from build123d import *

# Parameters (mm, degrees)
F0_W     = 50.8
F0_H     = 38.1
F1_DEPTH = 25.4
F3_DEPTH = 50.8
F4_W     = 19.05
F4_H     = 12.7
F5_DEPTH = 19.05


with BuildPart() as f1:
    # F0 (on Front) → F1 (new body)
    with BuildSketch(Plane.XZ):
        with Locations((16.882635, 19.05)):
            Rectangle(F0_W, F0_H)
    extrude(amount=F1_DEPTH)

    # F2 (on face) → F3 (cut)
    with BuildSketch(Plane.YZ.offset(42.282635)):
        with BuildLine():
            Line((-25.4, 38.1), (-25.4, 12.7))
            ThreePointArc((-25.4, 12.7), (-13.381807, 23.530105), (-6.35, 38.1))
            Line((-6.35, 38.1), (-25.4, 38.1))
        make_face()
    extrude(amount=-F3_DEPTH, mode=Mode.SUBTRACT)

    # F4 (on face) → F5 (cut)
    with BuildSketch(Plane.XY.offset(38.1)):
        with Locations((16.705383, -6.35)):
            Rectangle(F4_W, F4_H)
    extrude(amount=-F5_DEPTH, mode=Mode.SUBTRACT)


solid = f1.part
Model file for the job. Use its own axes, mm. A direction names the side the tool comes from. Give positions to 0.01 mm unless a question says otherwise; leave off trailing zeros. Loops run counter-clockwise (first coordinate to the right, second up) from the corner with the lowest first, then second, coordinate; pieces in that order, holes last.
1) Saw through at C-C (x = 38). Write the cut outline in (y, z).
2) Tool access for faces 5 (the flat face through (7.18, -5, 27)), 6 (the flat face through (17, -13, 0)): list every direction of +Z, -Z, +X, -X, +Y, -Y with a clear straight run to the whole face (end or side of a thin tool).
3) Wall check: line 1 (X direction, y = -2, z = 23); line 2 (Z direction, x = 21, y = -1.5); line 3 (Z direction, x = 13.5, y = -13.5). Give the ranges that are in metal, low to high.
4) Pull direction X, two halves, no side cores. Call faces 1 (the flat face through (17, -12.7, 22)), 2 (the flat face through (42.283, -10, 15)), 3 (the flat face through (-8.517, -10, 15)), 4 (the flat face through (34, -3, 38.1)): +X half, -X half, draft (parallel to the pull), parting line (faces both ways), or undercut.
5) Saw through at A-A (z = 29.5). Write the cut outline in (x, y), plus the area to 3 significant figures.
6) Saw through at B-B (y = -5). Write the cut outline in (x, z), plus the area to 3 significant figures.
7) Saw through at D-D (z = 22.5). Write the cut outline in (x, y).
8) Flat gauge pins, fed straight in: pin 1 Ø1 at (x, z) = (14.5, 26.5) entering from -Y; pin 2 Ø10 at (x, z) = (6, 33.5) entering from -Y; pin 3 Ø3 at (x, y) = (-1, -15) entering from +Z; pin 4 Ø10 at (x, y) = (33, -16) entering from +Z. Where does each tip first touch, or does it go through?
Answer block:
1. outline: (-25.4, 0) - (0, 0) - (0, 38.1) - (-6.35, 38.1) arc R41.99 cw to (-25.4, 12.7) - close
2. face 5: +Z, +Y
2. face 6: -Z, +X, -X, +Y, -Y
3. line 1: x = -8.52 to 7.18, 26.23 to 42.28
3. line 2: z = 0 to 19.05
3. line 3: z = 0 to 23.37
4. face 1: undercut
4. face 2: +X half
4. face 3: -X half
4. face 4: draft
5. outline: (-8.52, -9.64) - (7.18, -9.64) - (7.18, 0) - (-8.52, 0) - close; (26.23, -9.64) - (42.28, -9.64) - (42.28, 0) - (26.23, 0) - close
5. area: 306 mm2
6. outline: (-8.52, 0) - (42.28, 0) - (42.28, 38.1) - (26.23, 38.1) - (26.23, 19.05) - (7.18, 19.05) - (7.18, 38.1) - (-8.52, 38.1) - close
6. area: 1,570 mm2
7. outline: (-8.52, -14.18) - (42.28, -14.18) - (42.28, 0) - (26.23, 0) - (26.23, -12.7) - (7.18, -12.7) - (7.18, 0) - (-8.52, 0) - close
8. pin 1: passes through
8. pin 2: stops at y = -10.18
8. pin 3: stops at z = 23.37
8. pin 4: stops at z = 27.07
